Model file for the job. Use its own axes, mm. Give positions to 0.01 mm unless a question says otherwise; leave off trailing zeros. Loops run counter-clockwise (first coordinate to the right, second up) from the corner with the lowest first, then second, coordinate; pieces in that order, holes last. Notation, with made-up numbers: (29.25, 14) - (66.25, 14) arc R25 ccw to (66.25, 45) - close; hole circle Ø10 at (-21.5, -30). An arc over 180 degrees is marked (long way). Use a Markdown table: item, result.
from build123d import *

# Parameters (mm, degrees)
SKETCH1_W           = 36.83
SKETCH1_H           = 5.08
SKETCH1_W_2         = 25.4
BOSS_EXTRUDE1_DEPTH = 5.08
SKETCH2_W           = 5.08
SKETCH2_H           = 25.4
BOSS_EXTRUDE2_DEPTH = 5.08


with BuildPart() as part:
    # Sketch1 → Boss-Extrude1 (new body)
    with BuildSketch(Plane.XY):
        Polygon((59.69, -83.82), (96.52, -83.82), (96.52, 63.5), (59.69, 63.5), (34.29, 63.5), (-34.29, 63.5), (-59.69, 63.5), (-96.52, 63.5), (-96.52, -83.82), (-59.69, -83.82), (-34.29, -83.82), (-34.29, -88.9), (34.29, -88.9), (34.29, -83.82), align=None)
        with Locations((78.105, -86.36)):
            Rectangle(SKETCH1_W, SKETCH1_H)
        with Locations((-78.105, -86.36)):
            Rectangle(SKETCH1_W, SKETCH1_H)
        with Locations((46.99, 66.04)):
            Rectangle(SKETCH1_W_2, SKETCH1_H)
        with Locations((-46.99, 66.04)):
            Rectangle(SKETCH1_W_2, SKETCH1_H)
    extrude(amount=BOSS_EXTRUDE1_DEPTH)

    # Sketch2 → Boss-Extrude2 (add)
    with BuildSketch(Plane.XY.offset(5.08)):
        with Locations((99.06, -50.8)):
            Rectangle(SKETCH2_W, SKETCH2_H)
        with Locations((99.06, 30.48)):
            Rectangle(SKETCH2_W, SKETCH2_H)
        with Locations((-99.06, -50.8)):
            Rectangle(SKETCH2_W, SKETCH2_H)
        with Locations((-99.06, 30.48)):
            Rectangle(SKETCH2_W, SKETCH2_H)
    extrude(amount=-BOSS_EXTRUDE2_DEPTH)


solid = part.part
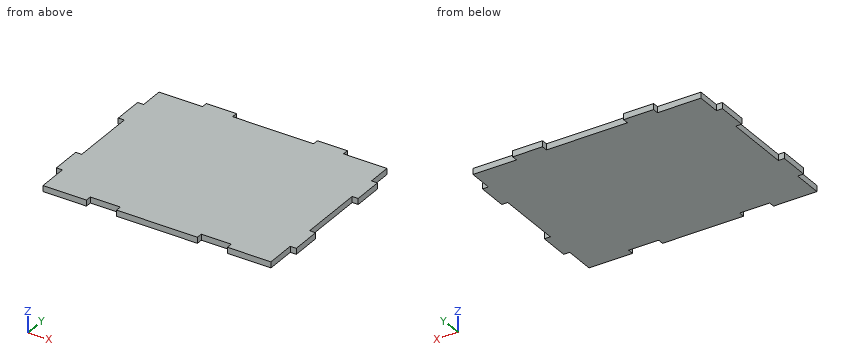
(1) Slice it at A-A, the plane x = 11.5. Write the cut outline in (y, z), plus the area to 3 significant figures.
Computed:
| item | result |
|---|---|
| outline | (-88.9, 0) - (63.5, 0) - (63.5, 5.08) - (-88.9, 5.08) - close |
| area | 774 mm² |
(2) Drill centre lines: probe 1 along X at (y, z) = (-1.5, 1.9); probe 2 along Y at (x, z) = (23, 1.8); probe 3 along Y at (x, z) = (40, 1.65). Where is each one in solid material? Low to high. Write a range as [from, to].
Computed:
| item | result |
|---|---|
| probe 1 | [-96.52, 96.52] |
| probe 2 | [-88.9, 63.5] |
| probe 3 | [-83.82, 68.58] |
(3) Pin check, flat tips, straight feed: P1, Ø2.5, axis at x = 99, z = 2.5, coming from the +Y side; P2, Ø12, axis at x = -55, y = 31.5, coming from the -Z side; P3, Ø2.5, axis at y = 66, z = 3.5, coming from the -X side; P4, Ø2.5, axis at x = -98.5, z = 3.5, coming from the -Y side. Stop position of each tip, or through.
Computed:
| item | result |
|---|---|
| P1 | y = 43.18 |
| P2 | z = 0 |
| P3 | x = -59.69 |
| P4 | y = -63.5 |
(4) Slice it at B-B, the plane y = 1.5. Write the cut outline in (x, z).
Computed:
| item | result |
|---|---|
| outline | (-96.52, 0) - (96.52, 0) - (96.52, 5.08) - (-96.52, 5.08) - close |
